Input: part model. Units: mm. Frame: model coordinates. Face numbers are marked on the shaded views. A direction names the side the tool comes from. Give positions to 0.01 mm unless a question says otherwise; leave off trailing zeros. Loops run counter-clockwise (first coordinate to the right, second up) from the corner with the lowest first, then second, coordinate; pieces in that order, holes last. Notation, with made-up numbers: (53.25, 1) -> (102.25, 1) arc R23 ccw to (102.25, 11) -> close; hole circle Ø1 at (51.5, 9). An arc over 180 degrees is marked (long way). Answer as a JSON object with one key per item and string values.
```python
from build123d import *

# Parameters (mm, degrees)
EXTRUDE_THIN1_DEPTH = 31
SKETCH6_R           = 3.5
CUT_EXTRUDE1_DEPTH  = 10
SKETCH7_R           = 3.302
CUT_EXTRUDE3_DEPTH  = 10.16


with BuildPart() as part:
    # Sketch1 → Extrude-Thin1 (new body)
    with BuildSketch(Plane(origin=(0, 0, 0), x_dir=(0, 0, -1), z_dir=(1, 0, 0))):
        Polygon((0, 0), (30, 0), (30, -29.972), (180, -29.972), (180, -39.972), (20, -39.972), (20, -10), (0, -10), align=None)
    extrude(amount=EXTRUDE_THIN1_DEPTH)

    # Sketch6 → Cut-Extrude1 (cut)
    with BuildSketch(Plane(origin=(0, 0, 0), x_dir=(1, 0, 0), z_dir=(0, 1, 0))):
        with Locations(Location((15.5, 15, 0), (0, 0, 270))):
            Circle(SKETCH6_R)
    extrude(amount=-CUT_EXTRUDE1_DEPTH, mode=Mode.SUBTRACT)

    # Sketch7 → Cut-Extrude3 (cut)
    with BuildSketch(Plane(origin=(0, -29.972, 0), x_dir=(1, 0, 0), z_dir=(0, 1, 0))):
        with Locations(Location((15.494, 158.524, 0), (0, 0, 270))):
            Circle(SKETCH7_R)
    extrude(amount=-CUT_EXTRUDE3_DEPTH, mode=Mode.SUBTRACT)


solid = part.part
```
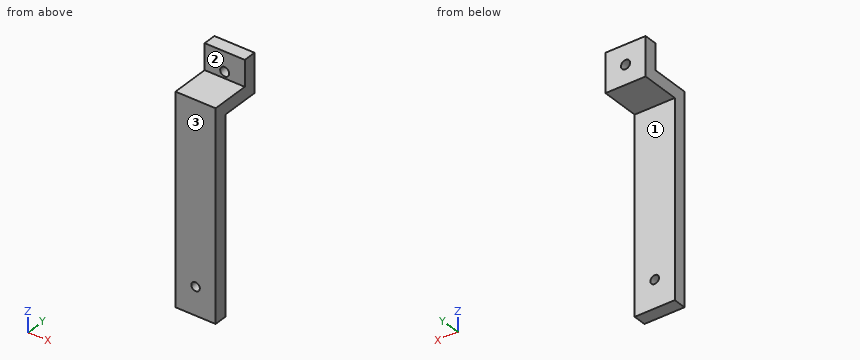
Q1. Section C-C, the plane x = 10.5. Return the cut outline in (y, z).
Evaluation:
{"outline": "(-39.97, -180) -> (-29.97, -180) -> (-29.97, -30) -> (0, -30) -> (0, 0) -> (-10, 0) -> (-10, -20) -> (-39.97, -20) -> close"}
Q2. Section D-D, the plane z = -146.5. Return the cut outline in (x, y).
Evaluation:
{"outline": "(0, -39.97) -> (31, -39.97) -> (31, -29.97) -> (0, -29.97) -> close"}
Q3. Ray query, line 1 along X through (y, z) = (-2.25, -15); line 2 along Z through (x, y) = (15, -7); line 3 along Y through (x, z) = (17, -113). Return the intervals inside material, ascending.
Evaluation:
{"line 1": "x = 0 to 12, 19 to 31", "line 2": "z = -30 to -18.46, -11.54 to 0", "line 3": "y = -39.97 to -29.97"}
Q4. Access query for the marked faces 1, 2 and 3. Directions: +Z, -Z, +X, -X, +Y, -Y. A direction counts if a zero-diameter tool reaches every point of the face in a straight line with its end or side. Return the directions, or none.
Evaluation:
{"face 1": "-Z, +X, -X, +Y", "face 2": "+Z, +X, -X, -Y", "face 3": "+Z, -Z, +X, -X, -Y"}
Q5. Pin query (flat end, axial travel): pin 1 (7.5 mm diameter, centred on x = 15.494, z = -158.524, fed in from -Y); pin 2 (1.5 mm diameter, centred on x = 19, y = -27, fed in from -Z); pin 3 (15 mm diameter, centred on x = 11.5, y = -19, fed in from +Z). Return the tip coordinate at first contact, or that it passes through.
Evaluation:
{"pin 1": "stops at y = -39.97", "pin 2": "stops at z = -30", "pin 3": "stops at z = -20"}
Q6. Section B-B, the plane y = -4. Return the cut outline in (x, z), then the cut area to 3 significant figures.
Evaluation:
{"outline": "(0, -30) -> (31, -30) -> (31, 0) -> (0, 0) -> close; hole circle Ø7 at (15.5, -15)", "area": "892 mm2"}
Q7. Section A-A, the plane z = -15. Return the cut outline in (x, y).
Evaluation:
{"outline": "(0, -10) -> (12, -10) -> (12, 0) -> (0, 0) -> close; (19, -10) -> (31, -10) -> (31, 0) -> (19, 0) -> close"}
